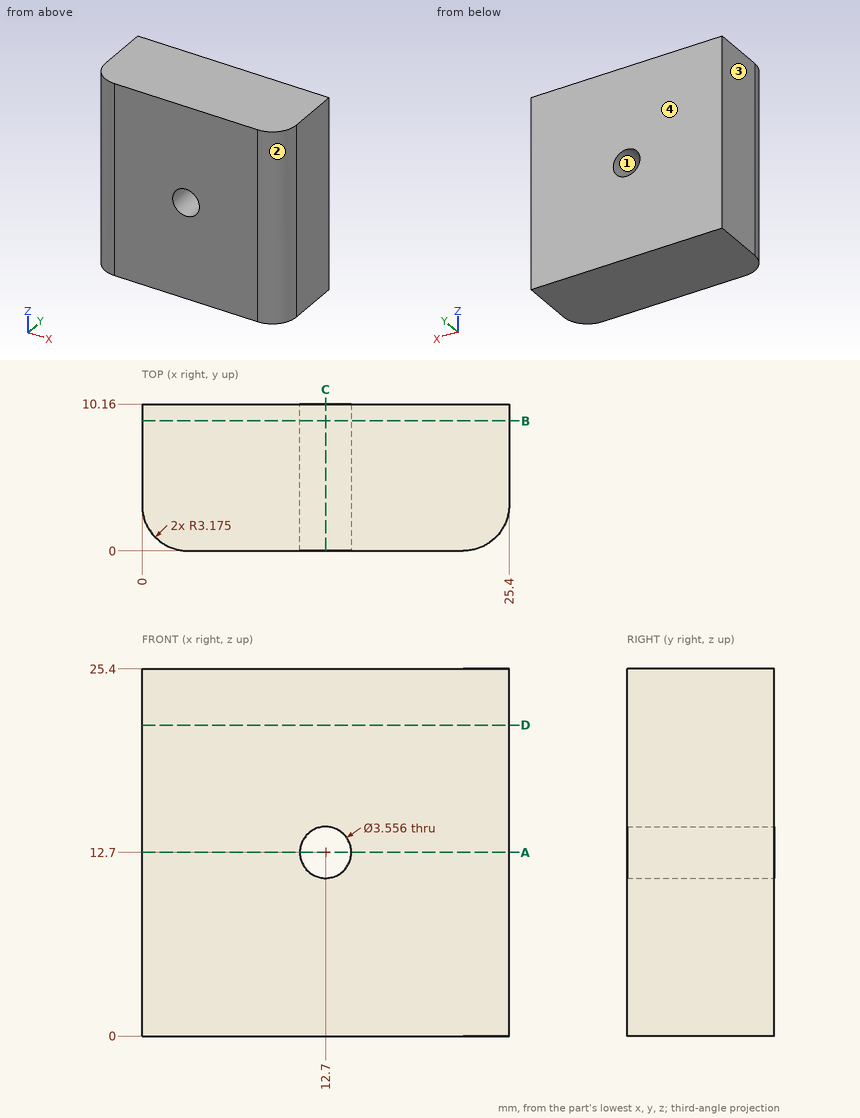
Can you work these out from the drawing? Everything is in mm from the part's minimum corner. Coordinates: 2 decimals unless noted, no trailing zeros. Loops run counter-clockwise (first coordinate to the right, second up) from the corner with the lowest first, then second, coordinate; pieces in that order, holes last.
1) Imagine slicing it at D-D on z = 21.5. List the corners of the cut face in (x, y) for me (3 decimals).
2) I need wall thicknesses on probe 1 along Z at (x, y) = (12.7, 3.25); probe 2 along X at (y, z) = (3.25, 12); probe 3 along Y at (x, z) = (22.75, 22). Which ranges of each line are inside material? Lowest first, please.
3) Thinking about a two-plate mould opening in X: for the marked faces 1, 2, 3 and 4, which applies, pulls with the +X half, pulls with the -X half, needs draft (parallel to the pull), parting line crosses it, or undercut?
4) Imagine slicing it at B-B on y = 9. List the corners of the cut face in (x, z) for me, plus the area to 3 significant figures.
5) Imagine slicing it at C-C on x = 12.7. List the corners of the cut face in (y, z) for me, plus the area to 3 significant figures.
6) Imagine slicing it at A-A on z = 12.7. List the corners of the cut face in (x, y) for me (3 decimals).
7) For pin 1 (2 mm diameter, centred on y = 1, z = 20.5, fed in from -X); pin 2 (3 mm diameter, centred on x = 12.7, z = 12.7, fed in from +Y), each with a flat end and sliding along its axis, tell me the tip position at first contact or that it passes through.
Completed:
1. outline: (0, 3.175) arc R3.175 ccw to (3.175, 0) - (22.225, 0) arc R3.175 ccw to (25.4, 3.175) - (25.4, 10.16) - (0, 10.16) - close
2. probe 1: z = 0 to 10.92, 14.48 to 25.4
2. probe 2: x = 0 to 11.07, 14.33 to 25.4
2. probe 3: y = 0.04 to 10.16
3. face 1: undercut
3. face 2: pulls with the +X half
3. face 3: pulls with the -X half
3. face 4: needs draft
4. outline: (0, 0) - (25.4, 0) - (25.4, 25.4) - (0, 25.4) - close; hole circle Ø3.56 at (12.7, 12.7)
4. area: 635 mm2
5. outline: (0, 0) - (10.16, 0) - (10.16, 10.92) - (0, 10.92) - close; (0, 14.48) - (10.16, 14.48) - (10.16, 25.4) - (0, 25.4) - close
5. area: 222 mm2
6. outline: (0, 3.175) arc R3.175 ccw to (3.175, 0) - (10.922, 0) - (10.922, 10.16) - (0, 10.16) - close; (14.478, 0) - (22.225, 0) arc R3.175 ccw to (25.4, 3.175) - (25.4, 10.16) - (14.478, 10.16) - close
7. pin 1: stops at x = 0.23
7. pin 2: passes through
